Read the model definition and answer for the solid it produces. Units are mm, in the model's axes. A direction names the side the tool comes from. Coordinates: 2 decimals unless noted, no trailing zeros. Write each loop counter-clockwise with the first axis right and the second up, starting at its lowest first coordinate (ties: lowest second). Pieces come first, ordered by that corner, then holes. Notation, with made-up numbers: (18, -21.5) - (25, -21.5) arc R11 cw to (25, -2.5) - close; hole circle Ø9 at (83, 62.5). An arc over 180 degrees is marked (long way). Use a Markdown table: item, result.
Autodesk Inventor part; units mm, degrees
ref_plane "YZ Plane" through (0, 0, 0) normal (1, 0, 0) x (0, 1, 0)
ref_plane "XZ Plane" through (0, 0, 0) normal (0, 1, 0) x (-1, 0, 0)
ref_plane "XY Plane" through (0, 0, 0) normal (0, 0, 1) x (1, 0, 0)
sketch "Sketch1" plane through (0, 0, 0) normal (0, 0, 1) x (1, 0, 0)
  line L0 (-9.677, -30.5907) -> (-13.477, -30.5907)
  line L1 (-9.677, -30.5907) -> (-9.677, -40.5907)
  line L2 (-9.677, -40.5907) -> (-11.677, -40.5907)
  line L3 (-11.677, -40.5907) -> (-11.677, -30.5907)
  line L4 (-9.677, -30.5907) -> (-9.677, -26.5988)
  line L5 (-13.477, -30.5907) -> (-13.477, -30.2107)
  line L6 (-13.477, -30.2107) -> (-13.477, -28.3907)
  line L7 (-13.477, -28.3907) -> (-9.677, -28.3907)
  point P0 (0, 0)
  dimension "d0" = 3.8
  dimension "d2" = 10
  dimension "d3" = 2
  dimension "d18" = 0.38
  dimension "d19" = 2.2
revolve "Revolution1" add sketch "Sketch1" angle 360 about axis through (-9.677, -30.5907, 0) along (0, -1, 0)
chamfer "Chamfer2" distance 0.2 angle 45 1 edges at (-7.677, -40.5907, 0)
thread "Rosca1"
fillet "Empalme2" radius 1.82 1 edges at (-5.877, -28.3907, 0)
sketch "Boceto2" plane through (-9.677, -28.3907, 0) normal (0, 1, 0) x (1, 0, 0)
  line L0 (1.1232, 0.9065) -> (1.3467, -0.5194)
  line L1 (1.3467, -0.5194) -> (0.2235, -1.426)
  line L2 (0.2235, -1.426) -> (-1.1232, -0.9065)
  line L3 (-1.1232, -0.9065) -> (-1.3467, 0.5194)
  line L4 (-1.3467, 0.5194) -> (-0.2235, 1.426)
  line L5 (-0.2235, 1.426) -> (1.1232, 0.9065)
  point P0 (9.677, 0)
  point P1 (0, 0)
  dimension "d21" = 2.5
extrude "Extrusión1" cut sketch "Boceto2" against normal blind 1.3
properties part number "Tornillo Allen cabeza botón M4x10mm"
(1) A cutting plane is placed at B-B, the plane y = -39.5. Write down the section's boundary in (x, z), and give its area (3 significant figures).
Report:
| item | result |
|---|---|
| outline | circle Ø4 at (-9.68, 0) |
| area | 12.6 mm² |
(2) The mould has two halves that part along Z. Classify faces 4 (the cylindrical face through (-7.68, -35.42, 0.09)), 5 (the flat face through (-10.12, -29.03, 1.17)), 6 (the flat face through (-8, -28.391, 0)): pulls with the +Z half, pulls with the -Z half, needs draft (parallel to the pull), parting line crosses it, or undercut.
Report:
| item | result |
|---|---|
| face 4 | parting line crosses it |
| face 5 | undercut |
| face 6 | needs draft |
(3) Straight lines are drawn through the part: L1, parallel to Z at x = -12.75, y = -30.5; L2, parallel to Y at x = -12.5, z = -0.25; L3, parallel to Z at x = -10, y = -32.5. For each, find the intervals that lie inside material, in ascending order.
Report:
| item | result |
|---|---|
| L1 | z = -2.24 to 2.24 |
| L2 | y = -30.59 to -28.6 |
| L3 | z = -1.97 to 1.97 |
(4) A cutting plane is placed at A-A, the plane z = 0. Write down the section's boundary in (x, y), and give its area (3 significant figures).
Report:
| item | result |
|---|---|
| outline | (-13.48, -30.59) - (-11.68, -30.59) - (-11.68, -40.39) - (-11.48, -40.59) - (-7.88, -40.59) - (-7.68, -40.39) - (-7.68, -30.59) - (-5.88, -30.59) - (-5.88, -30.21) arc R1.82 ccw to (-7.7, -28.39) - (-8.41, -28.39) - (-8.41, -29.69) - (-10.94, -29.69) - (-10.94, -28.39) - (-11.66, -28.39) arc R1.82 ccw to (-13.48, -30.21) - close |
| area | 52.0 mm² |
(5) For faces 1 (the flat face through (-10, -40.591, 0)), 2 (the flat face through (-10.47, -29.032, -0.966)), 3 (the flat face through (-11, -30.591, 2)), determine the directions among +Z, -Z, +X, -X, +Y, -Y from which every point of the face is accessible in a straight line to the end or side of a thin tool.
Report:
| item | result |
|---|---|
| face 1 | +Z, -Z, +X, -X, -Y |
| face 2 | +Y |
| face 3 | -Y |
(6) Each of these flat-tipped pins is pushed along its axis until it touches: P1, Ø2, axis at x = -12.5, z = 0.5, coming from the -Y side; P2, Ø1, axis at x = -9, y = -34.5, coming from the +Z side; P3, Ø4, axis at x = -7, y = -37.5, coming from the -Z side. Where does it stop, or does it pass through?
Report:
| item | result |
|---|---|
| P1 | stops at y = -40.52 |
| P2 | stops at z = 1.99 |
| P3 | stops at z = -1.88 |
